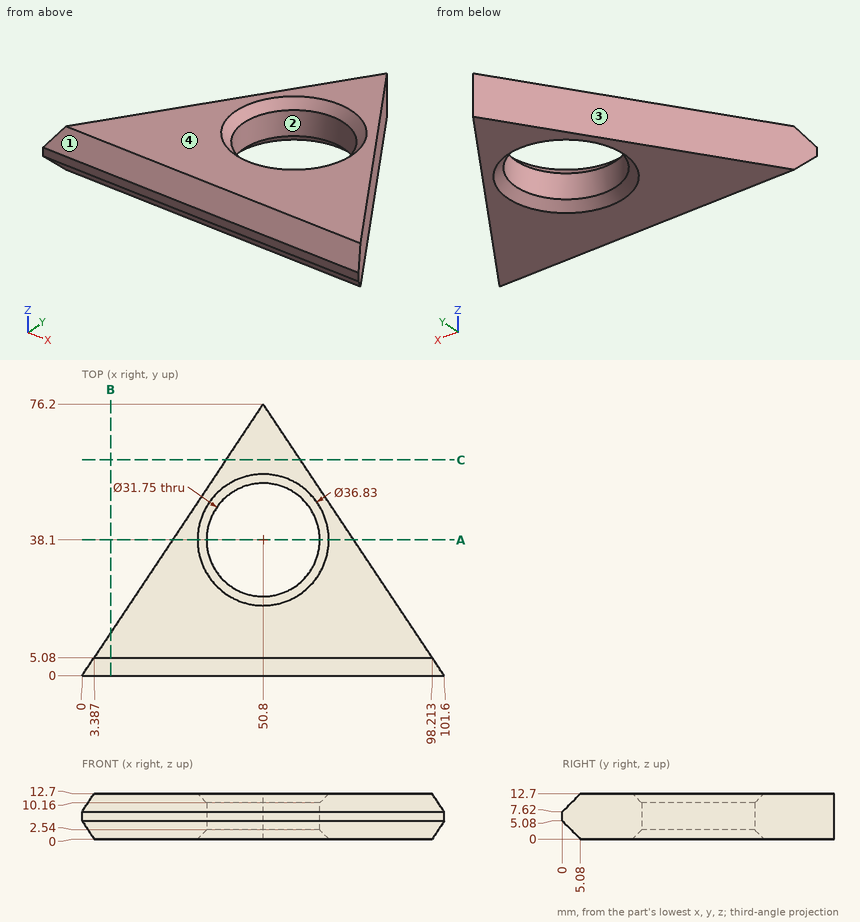
Drawing for the job (mm, zero at the part's lowest x, y, z). Give positions to 0.01 mm unless a question says otherwise; leave off trailing zeros. Loops run counter-clockwise (first coordinate to the right, second up) from the corner with the lowest first, then second, coordinate; pieces in that order, holes last. Notation, with made-up numbers: M 6,36.5 L 24,36.5 A23 cw 24,60.5 Z; hole C -7.5,15 d7. An arc over 180 degrees is marked long. Use one line per item in the form item = value.
Item 1: Slice it at B-B (x = 8). List the corners of the cut face in (y, z), plus the area to 3 significant figures.
Determined:
outline = M 0,5.08 L 5.08,0 L 12,0 L 12,12.7 L 5.08,12.7 L 0,7.62 Z
area = 127 mm2
Item 2: Two-plate mould, pull along Y, no slides. Class the marked faces 1, 2, 3 and 4: pulls with the +Y half, pulls with the -Y half, needs draft (parallel to the pull), parting line crosses it, or undercut.
Determined:
face_1 = pulls with the -Y half
face_2 = undercut
face_3 = pulls with the +Y half
face_4 = needs draft
Item 3: Drill centre lines: probe 1 along Y at (x, z) = (43.5, 0.5); probe 2 along X at (y, z) = (50.5, 10) (1 decimal); probe 3 along Y at (x, z) = (42, 6) (1 decimal). Where is each one in solid material? Low to high. Write a range as from..to.
Determined:
probe_1 = 4.58..21.74, 54.46..65.25
probe_2 = 33.7..40.9, 60.7..67.9
probe_3 = 0..24.9, 51.3..63
Item 4: Flat gauge pin, fed straight in: pin 1 (6 mm diameter, centred on x = 60.5, z = 4.5, fed in from -Y). Where does the tip first touch, or does it go through?
Determined:
pin_1 = 0
Item 5: Slice it at C-C (y = 60.5). List the corners of the cut face in (x, z).
Determined:
outline = M 40.33,0 L 61.27,0 L 61.27,12.7 L 40.33,12.7 Z
Item 6: Slice it at A-A (y = 38.1). List the corners of the cut face in (x, z) (1 decimal), plus the area to 3 significant figures.
Determined:
outline = M 25.4,0 L 32.4,0 L 34.9,2.5 L 34.9,10.2 L 32.4,12.7 L 25.4,12.7 Z; M 66.7,2.5 L 69.2,0 L 76.2,0 L 76.2,12.7 L 69.2,12.7 L 66.7,10.2 Z
area = 229 mm2
